Work out the finished part from the listing and answer in its coordinate system (mm). A direction names the side the tool comes from. Give positions to 0.01 mm unless a question says otherwise; leave off trailing zeros. Write each loop counter-clockwise with the first axis right and the second up, starting at its lowest first coordinate (ties: lowest second). Pieces come first, ordered by that corner, then holes. Notation, with made-up numbers: (-2, 88) - (25, 88) arc R30 cw to (25, 112) - close; hole circle Ø6 at (63, -37.75). An arc over 180 degrees is marked (long way). Write item = value, one per line.
from build123d import *

# Parameters (mm, degrees)
PAD003_DEPTH    = 1.49
PAD004_DEPTH    = 0.7
POCKET003_DEPTH = 0.75
CHAMFER_SIZE    = 0.08
PAD006_DEPTH    = 0.6
POCKET004_DEPTH = 7.456
SKETCH014_R     = 0.25
PAD007_DEPTH    = 0.68
FILLET002_R     = 0.1


with BuildPart() as part:
    # Sketch006 → Pad003 (new body)
    with BuildSketch(Plane.XZ.offset(-7.3)):
        with BuildLine():
            Line((0.3, 0), (0.3, 1.86))
            ThreePointArc((1.3, 2.86), (0.592893, 2.567107), (0.3, 1.86))
            Line((1.3, 2.86), (7.65, 2.86))
            ThreePointArc((8.65, 1.86), (8.357107, 2.567107), (7.65, 2.86))
            Line((8.65, 1.86), (8.65, 0))
            Line((8.65, 0), (0.3, 0))
        make_face()
    extrude(amount=PAD003_DEPTH)

    # Sketch008 → Pad004 (join)
    with BuildSketch(Plane.XZ.offset(-7.3)):
        with BuildLine():
            Line((0.78, 3.05147), (0.9, 2.776515))
            Line((0.9, 1.725), (0.9, 2.776515))
            Line((0.9, 1.725), (0, 1.725))
            Line((0, 1.725), (0, 1.86))
            ThreePointArc((0.78, 3.05147), (0.212342, 2.572039), (0, 1.86))
        make_face()
        with BuildLine():
            Line((8.05, 2.776515), (8.17, 3.05147))
            ThreePointArc((8.95, 1.86), (8.737658, 2.572039), (8.17, 3.05147))
            Line((8.95, 1.725), (8.95, 1.86))
            Line((8.05, 1.725), (8.95, 1.725))
            Line((8.05, 2.776515), (8.05, 1.725))
        make_face()
    extrude(amount=PAD004_DEPTH)

    # Sketch009 → Pocket003 (cut)
    with BuildSketch(Plane.XZ.offset(-7.3)):
        Polygon((2.17, 2.86), (2.17, 2.36), (2.575, 2.36), (3.075, 2.86), align=None)
        Polygon((5.875, 2.86), (6.375, 2.36), (6.78, 2.36), (6.78, 2.86), align=None)
    extrude(amount=POCKET003_DEPTH, mode=Mode.SUBTRACT)

    # Chamfer
    chamfer_edges = [part.edges().sort_by_distance(p)[0] for p in [
        (8.95, 6.6, 1.7925),
        (8.737658, 6.6, 2.572039),
        (8.17, 6.95, 3.05147),
        (6.78, 6.925, 2.86),
        (6.3275, 6.55, 2.86),
        (5.875, 6.925, 2.86),
        (3.075, 6.925, 2.86),
        (2.6225, 6.55, 2.86),
        (2.17, 6.925, 2.86),
        (0.78, 6.95, 3.05147),
        (0.212342, 6.6, 2.572039),
        (0, 6.6, 1.7925),
        (8.95, 6.95, 1.725),
        (0, 6.95, 1.725),
    ]]
    chamfer(chamfer_edges, length=CHAMFER_SIZE)

    # Sketch012 → Pad006 (join)
    with BuildSketch(Plane.XY.offset(1.28)):
        Polygon((1.495, 5.81), (1.495, 1.569294), (1.775, 0.8), (7.175, 0.8), (7.455, 1.569294), (7.455, 5.81), align=None)
    extrude(amount=PAD006_DEPTH)

    # Sketch013 → Pocket004 (cut, through all)
    with BuildSketch(Plane(origin=(1.495, 0.8, 1.88), x_dir=(0, 1, 0), z_dir=(1, 0, 0))):
        Polygon((0, -0.105), (0.181865, 0), (0, 0), align=None)
        Polygon((0, -0.6), (0.181865, -0.6), (0, -0.495), align=None)
    extrude(amount=POCKET004_DEPTH, mode=Mode.SUBTRACT)

    # Sketch014 → Pad007 (join)
    with BuildSketch(Plane.XY):
        with Locations((1.58, 6.25)):
            Circle(SKETCH014_R)
        with Locations((7.36, 6.25)):
            Circle(SKETCH014_R)
    extrude(amount=-PAD007_DEPTH)

    # Fillet002
    fillet002_edges = [part.edges().sort_by_distance(p)[0] for p in [
        (7.11, 6.25, -0.68),
        (1.33, 6.25, -0.68),
    ]]
    fillet(fillet002_edges, radius=FILLET002_R)


solid = part.part
1. Find section B-B, the plane x = 7.36. Give the vertices of the cut face in (y, z).
Solution:
outline = (1.31, 1.28) - (5.81, 1.28) - (5.81, 0) - (6, 0) - (6, -0.58) arc R0.1 ccw to (6.1, -0.68) - (6.4, -0.68) arc R0.1 ccw to (6.5, -0.58) - (6.5, 0) - (7.3, 0) - (7.3, 2.86) - (5.81, 2.86) - (5.81, 1.88) - (1.31, 1.88) - close
2. Find section D-D, the plane z = 0.45. Give the vertices of the cut face in (x, y).
Solution:
outline = (0.3, 5.81) - (8.65, 5.81) - (8.65, 7.3) - (0.3, 7.3) - close
3. A tool of negligible diameter and unlimited length cuts with its end or side. For faces 1 (the flat face through (4, 6, 2.86)), 2 (the flat face through (4, 3, 1.88)), 3 (the cylindrical face through (0.74, 6.4, 2.69)), 4 (the flat face through (5, 7.3, 1)), from which of +Z, -Z, +X, -X, +Y, -Y can it reach the whole face along a straight path? Write none if from no direction.
Solution:
face_1 = +Z, +Y, -Y
face_2 = +Z, +X, -X, -Y
face_3 = +Z, -Y
face_4 = +Z, -Z, +X, -X, +Y
4. Find section C-C, the plane z = -0.4. Give the vertices of the cut face in (x, y).
Solution:
outline = circle Ø0.5 at (1.58, 6.25); circle Ø0.5 at (7.36, 6.25)
5. For a pull along X with two mould halves and no side action, classify faces 5 (the flat face through (5, 7, 0)), 6 (the flat face through (4, 3, 1.28)), 7 (the cylindrical face through (8.233, 6.4, 2.673)) as pulls with the +X half, pulls with the -X half, needs draft (parallel to the pull), parting line crosses it, or undercut.
Solution:
face_5 = undercut
face_6 = needs draft
face_7 = undercut
6. Straight lines are drawn through the part: line 1 (Z direction, x = 4, y = 3.5); line 2 (X direction, y = 4.5, z = 1.55) (3 decimals); line 3 (Y direction, x = 2.75, z = 2.15). For each, find the intervals that lie inside material, in ascending order.
Solution:
line_1 = 1.28 to 1.88
line_2 = 1.495 to 7.455
line_3 = 5.81 to 7.3
7. Given pin 1 (1.5 mm diameter, centred on x = 2.5, z = 2, fed in from -Y); pin 2 (1.6 mm diameter, centred on y = 6.5, z = 0.5, fed in from +X); pin 3 (2 mm diameter, centred on y = 1.5, z = 1, fed in from +X) (3 decimals); pin 4 (0.5 mm diameter, centred on y = 7, z = 2.5, fed in from +X), each flat-ended and moving along its own axis, determine where each tip first touches the part or whether it passes through.
Solution:
pin_1 = 0.8
pin_2 = 8.65
pin_3 = 7.455
pin_4 = 8.89
8. Find section A-A, the plane y = 6.25. Give the vertices of the cut face in (x, z).
Solution:
outline = (0.3, 0) - (1.33, 0) - (1.33, -0.58) arc R0.1 ccw to (1.43, -0.68) - (1.73, -0.68) arc R0.1 ccw to (1.83, -0.58) - (1.83, 0) - (7.11, 0) - (7.11, -0.58) arc R0.1 ccw to (7.21, -0.68) - (7.51, -0.68) arc R0.1 ccw to (7.61, -0.58) - (7.61, 0) - (8.65, 0) - (8.65, 1.86) arc R1 ccw to (7.65, 2.86) - (1.3, 2.86) arc R1 ccw to (0.3, 1.86) - close
